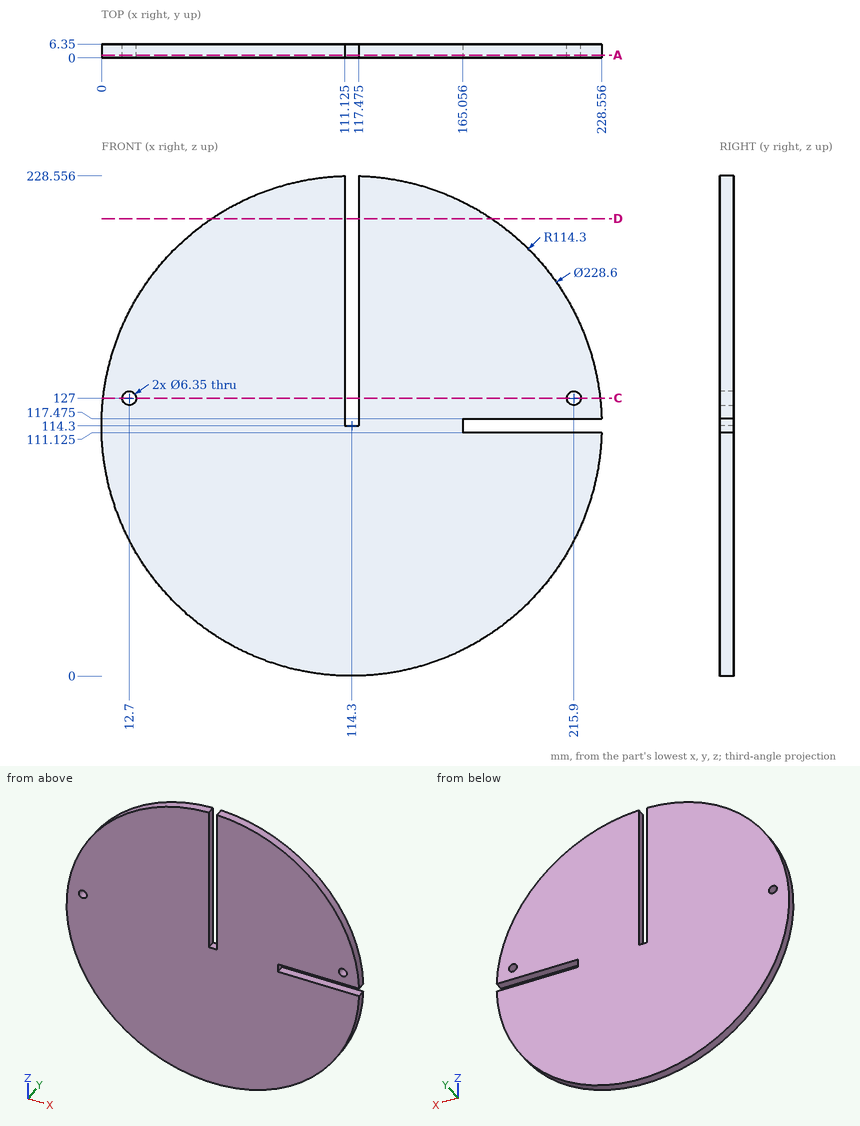
Verification items for this drawing (mm, ordinates from the low corner). Coordinates: 2 decimals unless noted, no trailing zeros. Write each loop counter-clockwise with the first axis right and the second up, starting at its lowest first coordinate (ties: lowest second). Pieces come first, ordered by that corner, then holes. Notation, with made-up numbers: (39, -11.75) - (59, -11.75) arc R19 cw to (59, 2.25) - close; hole circle Ø2 at (22.5, -20). An arc over 180 degrees is marked (long way). One line per question, with ' | ' between items.
Item 1: Sectioned sample at C-C on z = 127. Record the boundary of the cut face in (x, y) (3 decimals).
Determined:
outline: (0.708, 0) - (9.525, 0) - (9.525, 6.35) - (0.708, 6.35) - close; (15.875, 0) - (111.125, 0) - (111.125, 6.35) - (15.875, 6.35) - close; (117.475, 0) - (212.725, 0) - (212.725, 6.35) - (117.475, 6.35) - close; (219.075, 0) - (227.892, 0) - (227.892, 6.35) - (219.075, 6.35) - close
Item 2: Gauge pin test, flat ends, axial feed: P1, Ø3, axis at x = 115.5, y = 4, coming from the +Z side; P2, Ø1.5, axis at x = 182, y = 4, coming from the +Z side; P3, Ø3, axis at x = 54, y = 2, coming from the -Z side. Record the tip position at first contact, or that the pin passes through.
Determined:
P1: stops at z = 114.3 | P2: stops at z = 206.94 | P3: stops at z = 16.28
Item 3: Sectioned sample at A-A on y = 1.25. Record the boundary of the cut face in (x, z) (3 decimals).
Determined:
outline: (111.125, 114.3) - (111.125, 228.556) arc R114.3 ccw (long way) to (228.556, 111.125) - (165.056, 111.125) - (165.056, 117.475) - (228.556, 117.475) arc R114.3 ccw to (117.475, 228.556) - (117.475, 114.3) - close; hole circle Ø6.35 at (12.7, 127); hole circle Ø6.35 at (215.9, 127)
Item 4: Sectioned sample at D-D on z = 209. Record the boundary of the cut face in (x, y) (3 decimals).
Determined:
outline: (50.297, 0) - (111.125, 0) - (111.125, 6.35) - (50.297, 6.35) - close; (117.475, 0) - (178.303, 0) - (178.303, 6.35) - (117.475, 6.35) - close
Item 5: Thickness scan on line 1 (X direction, y = 5, z = 127) (1 decimal); line 2 (Z direction, x = 167, y = 2) (1 decimal); line 3 (X direction, y = 0.5, z = 144) (3 decimals). Record the ranges inside material, lowest first. Write a range as [from, to].
Determined:
line 1: x = [0.7, 9.5], [15.9, 111.1], [117.5, 212.7], [219.1, 227.9] | line 2: z = [12.9, 111.1], [117.5, 215.7] | line 3: x = [3.926, 111.125], [117.475, 224.674]
